```python
from build123d import *

# Parameters (mm, degrees)
BOSS_EXTRUDE1_DEPTH      = 40
BOSS_EXTRUDE1_DEPTH_BACK = 30
SKETCH1_W                = 70
SKETCH1_H                = 40
SKETCH1_R                = 10
CUT_EXTRUDE1_DEPTH       = 25
CUT_EXTRUDE1_DEPTH_BACK  = 25
SKETCH2_R                = 4.05
CUT_EXTRUDE2_START       = 40
SKETCH3_R                = 14.35
CUT_EXTRUDE2_DEPTH       = 8.1
CUT_EXTRUDE3_START       = -30
SKETCH4_R                = 14.2875
CUT_EXTRUDE3_DEPTH       = 8.1


with BuildPart() as part:
    # Sketch1 → Boss-Extrude1 (new, two sides: drawn at the far end of the back side and taken through both)
    with BuildSketch(Plane.XY.offset(-BOSS_EXTRUDE1_DEPTH_BACK)):
        Rectangle(SKETCH1_W, SKETCH1_H)
        Circle(SKETCH1_R, mode=Mode.SUBTRACT)
    extrude(amount=BOSS_EXTRUDE1_DEPTH + BOSS_EXTRUDE1_DEPTH_BACK)

    # Sketch2 → Cut-Extrude1 (cut, two sides: drawn at the far end of the back side and taken through both)
    with BuildSketch(Plane(origin=(0, 0, 0), x_dir=(1, 0, 0), z_dir=(0, 1, 0)).offset(-CUT_EXTRUDE1_DEPTH_BACK)):
        with Locations((-20, 20)):
            Circle(SKETCH2_R)
        with Locations((20, 20)):
            Circle(SKETCH2_R)
        with Locations((-20, -20)):
            Circle(SKETCH2_R)
        with Locations((20, -20)):
            Circle(SKETCH2_R)
        with Locations((-20, 0)):
            Circle(SKETCH2_R)
        with Locations((20, 0)):
            Circle(SKETCH2_R)
    extrude(amount=CUT_EXTRUDE1_DEPTH + CUT_EXTRUDE1_DEPTH_BACK, mode=Mode.SUBTRACT)

    # Sketch3 → Cut-Extrude2 (cut)
    with BuildSketch(Plane.XY.offset(CUT_EXTRUDE2_START)):
        Circle(SKETCH3_R)
    extrude(amount=-CUT_EXTRUDE2_DEPTH, mode=Mode.SUBTRACT)

    # Sketch4 → Cut-Extrude3 (cut)
    with BuildSketch(Plane.XY.offset(CUT_EXTRUDE3_START)):
        Circle(SKETCH4_R)
    extrude(amount=CUT_EXTRUDE3_DEPTH, mode=Mode.SUBTRACT)


solid = part.part
```
Model file for the job. Use its own axes, mm. A direction names the side the tool comes from. Coordinates: 2 decimals unless noted, no trailing zeros. Write each loop counter-clockwise with the first axis right and the second up, starting at its lowest first coordinate (ties: lowest second). Pieces come first, ordered by that corner, then holes. Notation, with made-up numbers: (-39, -13.75) - (17, -13.75) arc R11 ccw to (17, -0.75) - close; hole circle Ø6 at (-37.5, -31). An arc over 180 degrees is marked (long way). One line per question, with ' | ' between items. Start each with the question number.
Q1. Cut at B-B, the plane y = 5. List the corners of the cut face in (x, z), then the cut area to 3 significant figures.
Q2. Cut at C-C, the plane x = -7. List the corners of the cut face in (y, z), then the cut area to 3 significant figures.
Q3. Cut at A-A, the plane z = 0. List the corners of the cut face in (x, y), then the cut area to 3 significant figures.
Q4. Drill centre lines: line 1 (Z direction, x = 20, y = 6); line 2 (X direction, y = 0.5, z = -6.5); line 3 (Z direction, x = 18, y = -1). Where is each one in solid material? Low to high. Write a range as [from, to].
Q5. Cut at D-D, the plane z = -26. List the corners of the cut face in (x, y) (1 decimal), then the cut area to 3 significant figures.
Q6. 3-axis set-ups, long thin cutter, end or side, ignore diameter. For faces 1 (the face through (-10, -3, -21.9)), 2 (the face through (7.714, 12.1, 36.007)), 3 (the face through (7, 14, 40)): which of +Z, -Z, +X, -X, +Y, -Y reach the whole face in a straight line?
Q7. Pull direction Y, two halves, no side cores. Call faces 4 (the face through (0, 20, 5)), 5 (the face through (-35, 0, 5)), 6 (the face through (-14.274, 0.628, -26.007)): pulls with the +Y half, pulls with the -Y half, needs draft (parallel to the pull), parting line crosses it, or undercut.
Q8. Pin check, flat tips, straight feed: pin 1 (13 mm diameter, centred on x = -20, z = -20, fed in from +Y); pin 2 (5 mm diameter, centred on x = 8.5, y = -4.5, fed in from +Z); pin 3 (3 mm diameter, centred on x = 4.5, y = 6, fed in from -Z); pin 4 (8.5 mm diameter, centred on x = 7, y = -6.5, fed in from -Z). Stop position of each tip, or through.
Answer below:
1) outline: (-35, -30) - (-13.38, -30) - (-13.38, -21.9) - (-8.66, -21.9) - (-8.66, 31.9) - (-13.45, 31.9) - (-13.45, 40) - (-35, 40) - close; (8.66, -21.9) - (13.38, -21.9) - (13.38, -30) - (35, -30) - (35, 40) - (13.45, 40) - (13.45, 31.9) - (8.66, 31.9) - close; hole circle Ø8.1 at (-20, -20); hole circle Ø8.1 at (-20, 0); hole circle Ø8.1 at (-20, 20); hole circle Ø8.1 at (20, -20); hole circle Ø8.1 at (20, 0); hole circle Ø8.1 at (20, 20) | area: 3,220 mm^2
2) outline: (-20, -30) - (-12.46, -30) - (-12.46, -21.9) - (-7.14, -21.9) - (-7.14, 31.9) - (-12.53, 31.9) - (-12.53, 40) - (-20, 40) - close; (7.14, -21.9) - (12.46, -21.9) - (12.46, -30) - (20, -30) - (20, 40) - (12.53, 40) - (12.53, 31.9) - (7.14, 31.9) - close | area: 1,630 mm^2
3) outline: (-35, -20) - (-24.05, -20) - (-24.05, 20) - (-35, 20) - close; (-15.95, -20) - (15.95, -20) - (15.95, 20) - (-15.95, 20) - close; (24.05, -20) - (35, -20) - (35, 20) - (24.05, 20) - close; hole circle Ø20 at (0, 0) | area: 1,840 mm^2
4) line 1: [-30, -24.05], [-15.95, -4.05], [4.05, 15.95], [24.05, 40] | line 2: [-35, -9.99], [9.99, 35] | line 3: [-30, -23.52], [-16.48, -3.52], [3.52, 16.48], [23.52, 40]
5) outline: (-35, -20) - (35, -20) - (35, 20) - (-35, 20) - close; hole circle Ø28.6 at (0, 0) | area: 2,160 mm^2
6) face 1: -Z | face 2: +Z | face 3: +Z, +X, -X, +Y, -Y
7) face 4: pulls with the +Y half | face 5: needs draft | face 6: undercut
8) pin 1: y = 20 | pin 2: z = 31.9 | pin 3: through | pin 4: z = -21.9
